from build123d import *

# Parameters (mm, degrees)
SKETCH1_R           = 12
SKETCH1_R_2         = 3.05
BOSS_EXTRUDE1_DEPTH = 3
BOSS_EXTRUDE2_START = 10
SKETCH1_3_R         = 5
SKETCH1_3_R_2       = 3.05
BOSS_EXTRUDE2_DEPTH = 10
SKETCH2_R           = 1
CUT_EXTRUDE1_DEPTH  = 10


with BuildPart() as part:
    # Sketch1 → Boss-Extrude1 (new body)
    with BuildSketch(Plane(origin=(0, 0, 0), x_dir=(0, 0, -1), z_dir=(1, 0, 0))):
        Circle(SKETCH1_R)
        Circle(SKETCH1_R_2, mode=Mode.SUBTRACT)
    extrude(amount=-BOSS_EXTRUDE1_DEPTH)

    # Sketch1<3> → Boss-Extrude2 (add)
    with BuildSketch(Plane(origin=(0, 0, 0), x_dir=(0, 0, -1), z_dir=(1, 0, 0)).offset(BOSS_EXTRUDE2_START)):
        Circle(SKETCH1_3_R)
        Circle(SKETCH1_3_R_2, mode=Mode.SUBTRACT)
    extrude(amount=-BOSS_EXTRUDE2_DEPTH)

    # Sketch2 → Cut-Extrude1 (cut)
    with BuildSketch(Plane.ZY.offset(3)):
        with Locations((-6.01040764, 6.01040764)):
            Circle(SKETCH2_R)
        with Locations((-6.01040764, -6.01040764)):
            Circle(SKETCH2_R)
        with Locations((6.01040764, 6.01040764)):
            Circle(SKETCH2_R)
        with Locations((6.01040764, -6.01040764)):
            Circle(SKETCH2_R)
    extrude(amount=-CUT_EXTRUDE1_DEPTH, mode=Mode.SUBTRACT)


solid = part.part
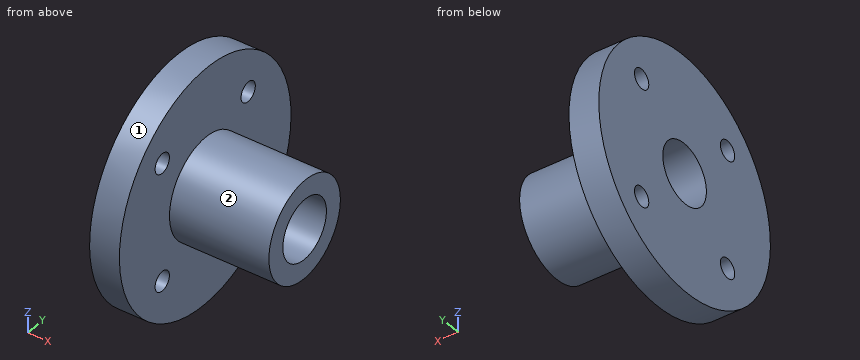
Could you check a few things on this model? Use its own coordinates, in mm. Face numbers are marked on the shaded views. A direction names the side the tool comes from. Give positions to 0.01 mm unless a question says otherwise; leave off trailing zeros. Order: outer loops, then holes, each group sorted by start corner. A loop starts at its lowest first (then second) coordinate and runs counter-clockwise, first axis right, second up. Notation, with made-up numbers: (0.5, -33.75) -> (20.5, -33.75) arc R13 ccw to (20.5, -28.75) -> close; hole circle Ø11 at (49.5, 19). An arc over 180 degrees is marked (long way). Answer in a Markdown table with one row per item. Add a question column.
Item 1: Imagine slicing it at A-A (z = 0). List the corners of the cut face in (x, y) for me.
Item 2: Imagine slicing it at C-C (z = 6). List the corners of the cut face in (x, y) for me.
Item 3: Please list where these lines run through material, in increasing order: probe 1 along Y at (x, z) = (-2, -5.25); probe 2 along Y at (x, z) = (4.25, -1); probe 3 along X at (y, z) = (-9.25, -2.25).
Item 4: I'm going to push flat-ended pins straight in: P1, Ø1.6, axis at y = 6.01, z = -6.01, coming from the -X side; P2, Ø2.5, axis at y = -6.01, z = 6.01, coming from the +X side; P3, Ø2.5, axis at y = -6.01, z = -6.01, coming from the -X side; P4, Ø4, axis at x = 3, y = 1, coming from the +Z side. Where does each tip first touch, or does it pass through?
Item 5: For the marked faces 1 and 2, which set-ups out of +Z, -Z, +X, -X, +Y, -Y let a thin tool reach every point of the face, with its end or its side?
Item 6: Imagine slicing it at D-D (x = -0.5). List the corners of the cut face in (y, z) for me, and give its area (3 significant figures).
Result:
| question | item | result |
|---|---|---|
| 1 | outline | (-3, -12) -> (0, -12) -> (0, -5) -> (10, -5) -> (10, -3.05) -> (-3, -3.05) -> close; (-3, 3.05) -> (10, 3.05) -> (10, 5) -> (0, 5) -> (0, 12) -> (-3, 12) -> close |
| 2 | outline | (-3, -10.39) -> (0, -10.39) -> (0, -7.01) -> (-3, -7.01) -> close; (-3, -5.01) -> (0, -5.01) -> (0, 5.01) -> (-3, 5.01) -> close; (-3, 7.01) -> (0, 7.01) -> (0, 10.39) -> (-3, 10.39) -> close |
| 3 | probe 1 | -10.79 to -6.66, -5.36 to 5.36, 6.66 to 10.79 |
| 3 | probe 2 | -4.9 to -2.88, 2.88 to 4.9 |
| 3 | probe 3 | -3 to 0 |
| 4 | P1 | through |
| 4 | P2 | x = 0 |
| 4 | P3 | x = -3 |
| 4 | P4 | z = 5 |
| 5 | face 1 | +X, -X |
| 5 | face 2 | +X |
| 6 | outline | circle Ø24 at (0, 0); hole circle Ø2 at (-6.01, -6.01); hole circle Ø2 at (-6.01, 6.01); hole circle Ø6.1 at (0, 0); hole circle Ø2 at (6.01, -6.01); hole circle Ø2 at (6.01, 6.01) |
| 6 | area | 411 mm2 |
